from build123d import *

# Parameters (mm, degrees)
F0_W      = 42.3
F0_H      = 42.3
F1_DEPTH  = 19.75
F2_SIZE   = 2.54
F4_D      = 3.3
F4_DEPTH  = 4.5
F4_TIP    = 0.9914200214
F5_R      = 18
F6_DEPTH  = 48.2
F7_R      = 11
F8_DEPTH  = 2
F9_R      = 4
F10_DEPTH = 18
F11_SIZE  = 1.27


with BuildPart() as f1:
    # F0 (on Front) → F1 (new body, symmetric)
    with BuildSketch(Plane.XZ):
        Rectangle(F0_W, F0_H)
    extrude(amount=F1_DEPTH, both=True)

    # F2
    f2_edges = [f1.edges().sort_by_distance(p)[0] for p in [
        (21.15, 0, 21.15),
        (-21.15, 0, 21.15),
        (-21.15, 0, -21.15),
        (21.15, 0, -21.15),
    ]]
    chamfer(f2_edges, length=F2_SIZE)

    # F4
    with Locations(Plane.XZ.offset(19.75)):
        with Locations((15.5, 15.5), (15.5, -15.5), (-15.5, -15.5), (-15.5, 15.5)):
            Hole(F4_D / 2, depth=F4_DEPTH)
            with Locations((0, 0, -(F4_DEPTH + F4_TIP / 2))):  # 118° drill point
                Cone(0, F4_D / 2, F4_TIP, mode=Mode.SUBTRACT)

    # F5 (on face) → F6 (join)
    with BuildSketch(Plane.XZ.offset(19.75)):
        Circle(F5_R)
    extrude(amount=F6_DEPTH)

    # F7 (on face) → F8 (join)
    with BuildSketch(Plane.XZ.offset(67.95)):
        Circle(F7_R)
    extrude(amount=F8_DEPTH)

    # F9 (on face) → F10 (join)
    with BuildSketch(Plane.XZ.offset(69.95)):
        Circle(F9_R)
    extrude(amount=F10_DEPTH)

    # F11
    f11_edges = [f1.edges().sort_by_distance(p)[0] for p in [
        (-18, -67.95, 0),
    ]]
    chamfer(f11_edges, length=F11_SIZE)


solid = f1.part
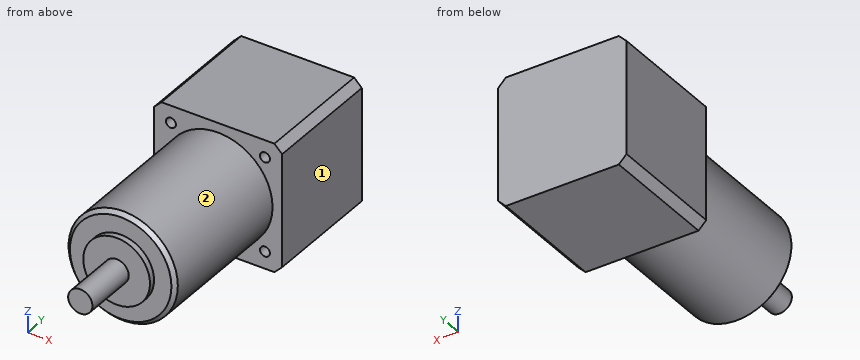
Read the model definition and answer for the solid it produces. Units are mm, in the model's axes. Face numbers are marked on the shaded views. A direction names the side the tool comes from. Give positions to 0.01 mm unless a question says otherwise; leave off trailing zeros. Write each loop counter-clockwise with the first axis right and the second up, starting at its lowest first coordinate (ties: lowest second). Pieces come first, ordered by that corner, then holes. Notation, with made-up numbers: (56, -12) - (81, -12) arc R21 cw to (81, 18) - close; hole circle Ø2 at (40.5, 11). An arc over 180 degrees is marked (long way). Answer in a Markdown table with one row per item. Add a question column.
Item 1: Section C-C, the plane y = -43 is taken. Write down the section's boundary in (x, z).
Item 2: A tool of negligible diameter and unlimited length cuts with its end or side. For the marked faces 1 and 2, from which of +Z, -Z, +X, -X, +Y, -Y can it reach the whole face along a straight path? Write none if from no direction.
Item 3: Section B-B, the plane z = 0 is taken. Write down the section's boundary in (x, y).
Item 4: Section A-A, the plane x = 0 is taken. Write down the section's boundary in (y, z).
Item 5: Flat-ended cylindrical pins translate along their axes: P1, Ø3, axis at x = 2, z = -6, coming from the -Y side; P2, Ø8, axis at y = -57, z = 11.5, coming from the -X side; P3, Ø4, axis at x = -15.5, z = 15.5, coming from the -Y side. Find the tip coordinate at first contact, or state that the pin passes through.
Item 6: Find the intervals of material crossed by L1, parallel to X at y = -17.75, z = -15.5; L2, parallel to Y at x = 7.5, z = 5, in increasing order.
Recorded:
| question | item | result |
|---|---|---|
| 1 | outline | circle Ø36 at (0, 0) |
| 2 | face 1 | +Z, -Z, +X, +Y, -Y |
| 2 | face 2 | -Y |
| 3 | outline | (-21.15, -19.75) - (-18, -19.75) - (-18, -66.68) - (-16.73, -67.95) - (-11, -67.95) - (-11, -69.95) - (-4, -69.95) - (-4, -87.95) - (4, -87.95) - (4, -69.95) - (11, -69.95) - (11, -67.95) - (16.73, -67.95) - (18, -66.68) - (18, -19.75) - (21.15, -19.75) - (21.15, 19.75) - (-21.15, 19.75) - close |
| 4 | outline | (-87.95, -4) - (-69.95, -4) - (-69.95, -11) - (-67.95, -11) - (-67.95, -16.73) - (-66.68, -18) - (-19.75, -18) - (-19.75, -21.15) - (19.75, -21.15) - (19.75, 21.15) - (-19.75, 21.15) - (-19.75, 18) - (-66.68, 18) - (-67.95, 16.73) - (-67.95, 11) - (-69.95, 11) - (-69.95, 4) - (-87.95, 4) - close |
| 5 | P1 | stops at y = -69.95 |
| 5 | P2 | stops at x = -16.36 |
| 5 | P3 | stops at y = -19.75 |
| 6 | L1 | x = -21.15 to -17.15, -13.85 to 13.85, 17.15 to 21.15 |
| 6 | L2 | y = -69.95 to 19.75 |
